Build history of the part. All positions in model axes, mm. Face numbers are marked on the shaded views. A direction names the side the tool comes from. Round coordinates to 2 decimals unless told otherwise and drop trailing zeros. Write each loop counter-clockwise with the first axis right and the second up, starting at its lowest first coordinate (ties: lowest second). Pieces come first, ordered by that corner, then holes.
1) Which spindle directions (+Z, -Z, +X, -X, +Y, -Y) get a long thin tool onto all of the face, cutting with end or side? Do the marked faces 4 and 5. Say none if no direction does.
2) Pull direction Z, two halves, no side cores. Call the marked faces 1, 2 and 3: +Z half, -Z half, draft (parallel to the pull), parting line (faces both ways), or undercut.
3) Saw through at C-C (y = 0.95). Write the cut outline in (x, z), plus the area to 3 significant figures.
4) Saw through at A-A (z = 3). Write the cut outline in (x, y).
5) Wall check: probe 1 along X at (y, z) = (0.2, 3.75); probe 2 along Z at (x, y) = (0.75, 0.45). Give the ranges that are in metal, low to high.
6) Saw through at B-B (x = -6). Write the cut outline in (y, z), plus the area to 3 significant figures.
7) Flat gauge pin, fed straight in: pin 1 (1.5 mm diameter, centred on x = -6, z = 2.5, fed in from -Y). Where does the tip first touch, or does it go through?
from build123d import *

# Parameters (mm, degrees)
SKETCH005_W      = 16.898421
SKETCH005_H      = 8
EXTRUDE004_DEPTH = 2.5
SKETCH_W         = 19
SKETCH_H         = 2
EXTRUDE_DEPTH    = 10


with BuildPart() as extrude004:
    # Sketch005 (on Face2 of Extrude) → Extrude004 (new body, symmetric)
    with BuildSketch(Plane.XZ):
        with Locations((0.05079, 5)):
            Rectangle(SKETCH005_W, SKETCH005_H)
    extrude(amount=EXTRUDE004_DEPTH, both=True)


with BuildPart() as cut001:
    # Sketch → Extrude (new body)
    with BuildSketch(Plane.XY):
        with Locations((0, 1)):
            Rectangle(SKETCH_W, SKETCH_H)
    extrude(amount=EXTRUDE_DEPTH)

    # Cut001: cut Extrude004
    add(extrude004.part, mode=Mode.SUBTRACT)


solid = cut001.part
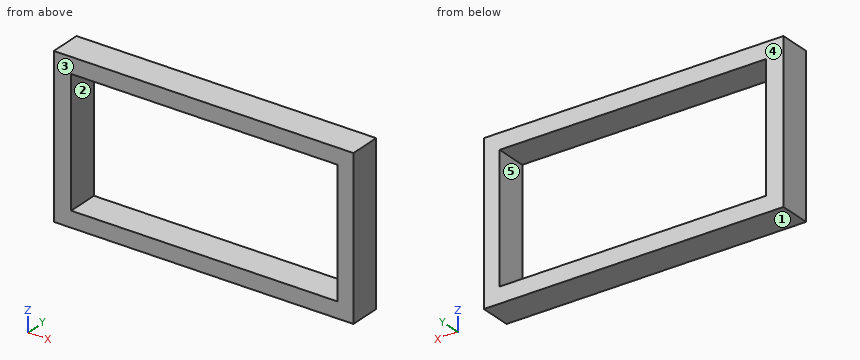
Evaluation:
1. face 4: +Z, -Z, +X, -X, +Y
1. face 5: +Y, -Y
2. face 1: -Z half
2. face 2: undercut
2. face 3: draft
3. outline: (-9.5, 0) - (9.5, 0) - (9.5, 10) - (-9.5, 10) - close; hole (-8.4, 1) - (8.5, 1) - (8.5, 9) - (-8.4, 9) - close
3. area: 54.8 mm2
4. outline: (-9.5, 0) - (-8.4, 0) - (-8.4, 2) - (-9.5, 2) - close; (8.5, 0) - (9.5, 0) - (9.5, 2) - (8.5, 2) - close
5. probe 1: x = -9.5 to -8.4, 8.5 to 9.5
5. probe 2: z = 0 to 1, 9 to 10
6. outline: (0, 0) - (2, 0) - (2, 1) - (0, 1) - close; (0, 9) - (2, 9) - (2, 10) - (0, 10) - close
6. area: 4.00 mm2
7. pin 1: passes through
